Design review of the part shown in the three views and the two pictorial views. Dimensions are in mm from the part's minimum x, y and z. A direction names the side the tool comes from. Round coordinates to 2 decimals unless told otherwise and drop trailing zeros. Loops run counter-clockwise (first coordinate to the right, second up) from the corner with the lowest first, then second, coordinate; pieces in that order, holes last.
1) Mouldability with a two-part tool opening along X and no side actions: class the marked faces 1, 2 and 3 as pulls with the +X half, pulls with the -X half, needs draft (parallel to the pull), parting line crosses it, or undercut.
2) Insertion check: pin 1 (1.2 mm diameter, centred on y = 1, z = 11, fed in from +X) (1 decimal); pin 2 (0.8 mm diameter, centred on y = 2, z = 11, fed in from -X); pin 3 (0.8 mm diameter, centred on x = 5.5, y = 1, fed in from +Z). Each pin has a flat end and moves straight along its axis. Give the tip position at first contact, or say it passes through.
3) Take a section at C-C (y = 1.85). State the section outline as (x, z) points, then the cut area to 3 significant figures.
4) Tool access review of the marked faces 4, 5 and 6: name each direction out of +Z, -Z, +X, -X, +Y, -Y from which nothing blocks a thin tool from reaching the whole face with its end or side.
5) Take a section at D-D (x = 15.75). State the section outline as (y, z) points.
6) Wall thickness on L1, parallel to X at y = 2.3, z = 5.5 (1 decimal); L2, parallel to X at y = 1.75, z = 9 (1 decimal); L3, parallel to X at y = 1.3, z = 11.75 (1 decimal): over which ranges is each line inside the solid? List them lowest first.
7) Take a section at A-A (z = 6.75). State the section outline as (x, y) points.
8) Take a section at B-B (z = 1.5). State the section outline as (x, y) points (1 decimal).
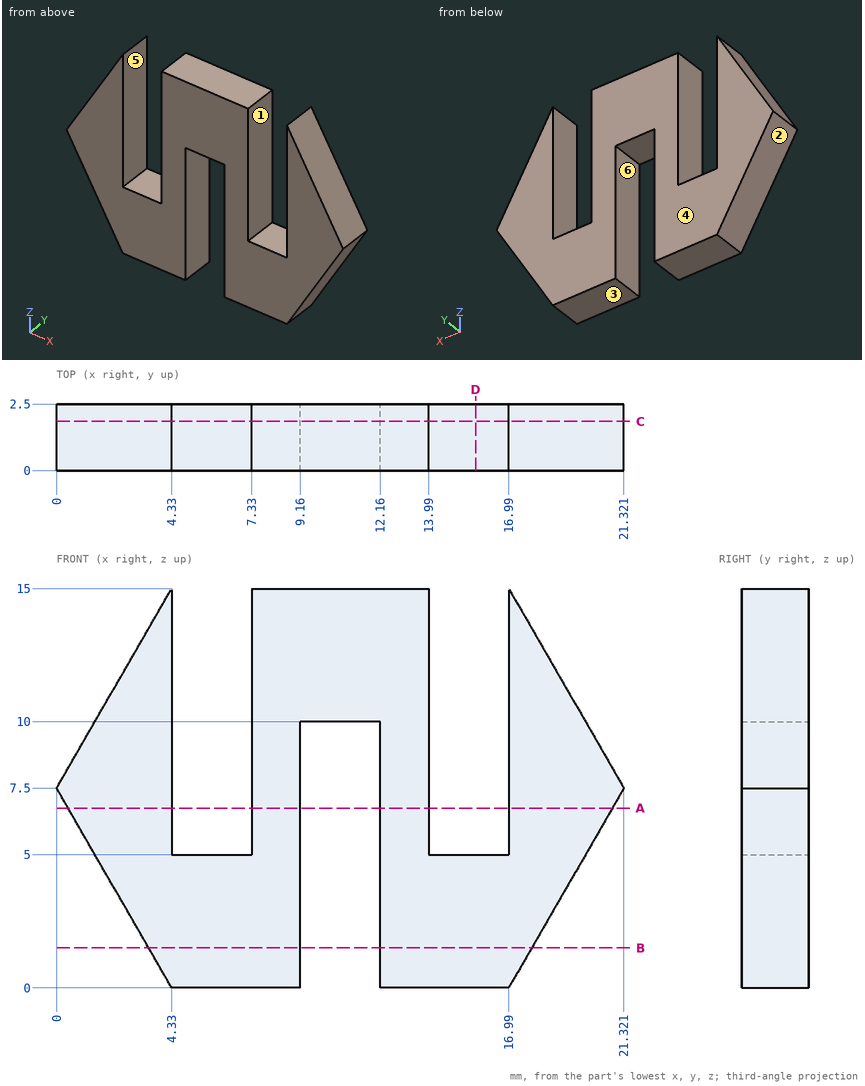
Response:
1. face 1: undercut
1. face 2: pulls with the -X half
1. face 3: needs draft
2. pin 1: stops at x = 19.6
2. pin 2: stops at x = 1.79
2. pin 3: stops at z = 5
3. outline: (0, 7.5) - (4.33, 0) - (9.16, 0) - (9.16, 10) - (12.16, 10) - (12.16, 0) - (16.99, 0) - (21.32, 7.5) - (16.99, 15) - (16.99, 5) - (13.99, 5) - (13.99, 15) - (7.33, 15) - (7.33, 5) - (4.33, 5) - (4.33, 15) - close
3. area: 165 mm2
4. face 4: +Z, -Z, +X, -X, +Y
4. face 5: +Z, +Y, -Y
4. face 6: -Z, +Y, -Y
5. outline: (0, 0) - (2.5, 0) - (2.5, 5) - (0, 5) - close
6. L1: x = 1.2 to 4.3, 7.3 to 9.2, 12.2 to 14, 17 to 20.2
6. L2: x = 0.9 to 4.3, 7.3 to 9.2, 12.2 to 14, 17 to 20.5
6. L3: x = 2.5 to 4.3, 7.3 to 14, 17 to 18.9
7. outline: (0.43, 0) - (4.33, 0) - (4.33, 2.5) - (0.43, 2.5) - close; (7.33, 0) - (9.16, 0) - (9.16, 2.5) - (7.33, 2.5) - close; (12.16, 0) - (13.99, 0) - (13.99, 2.5) - (12.16, 2.5) - close; (16.99, 0) - (20.89, 0) - (20.89, 2.5) - (16.99, 2.5) - close
8. outline: (3.5, 0) - (9.2, 0) - (9.2, 2.5) - (3.5, 2.5) - close; (12.2, 0) - (17.9, 0) - (17.9, 2.5) - (12.2, 2.5) - close
